```python
from build123d import *

# Parameters (mm, degrees)
BOSS_EXTRUDE1_DEPTH      = 3
BOSS_EXTRUDE1_DEPTH_BACK = 3
FILLET1_R                = 1


with BuildPart() as part:
    # Sketch2 → Boss-Extrude1 (new body, two sides)
    with BuildSketch(Plane(origin=(58.083917136, 121.431989422, 69.518693427), x_dir=(0.999322072, -0.036815702, 0), z_dir=(0, 0, 1))) as boss_extrude1_sk:
        with BuildLine():
            ThreePointArc((18.431354186, -334.485007307), (12.322654185, -340.593707309), (6.213954184, -334.485007307))
            Line((6.213954184, -334.485007307), (-8.62450673, -0.768484104))
            ThreePointArc((-8.62450673, -0.768484104), (-8.650130074, -0.384621702), (-8.658676813, 0))
            ThreePointArc((-8.658676813, 0), (0, 8.658676813), (8.658676813, 0))
            Line((8.658676813, 0), (21.001241455, -149.039780561))
            Line((21.001241455, -149.039780561), (21.131937197, -152.587373918))
            Line((21.131937197, -152.587373918), (18.13397098, -152.697821023))
            Line((18.13397098, -152.697821023), (18.003275238, -149.150227667))
            Line((18.003275238, -149.150227667), (17.003953166, -149.187043369))
            Line((17.003953166, -149.187043369), (17.17146461, -153.733958797))
            Line((17.17146461, -153.733958797), (22.168074971, -153.549880288))
            Line((22.168074971, -153.549880288), (22.00294469, -149.067598925))
            Line((22.00294469, -149.067598925), (9.66, 0))
            ThreePointArc((9.66, 0), (0, 9.66), (-9.66, 0))
            Line((-9.66, 0), (-9.621878236, -0.857355938))
            Line((-9.621878236, -0.857355938), (5.212654184, -334.485007307))
            ThreePointArc((5.212654184, -334.485007307), (12.322654185, -341.595007309), (19.432654186, -334.485007307))
            Line((19.432654186, -334.485007307), (24.411992001, -214.458560592))
            Line((24.411992001, -214.458560592), (24.244480558, -209.911645163))
            Line((24.244480558, -209.911645163), (19.247192269, -210.095748648))
            Line((19.247192269, -210.095748648), (19.414703712, -214.642664077))
            Line((19.414703712, -214.642664077), (20.414703712, -214.605823399))
            Line((20.414703712, -214.605823399), (20.284007971, -211.058230043))
            Line((20.284007971, -211.058230043), (23.281974187, -210.947782937))
            Line((23.281974187, -210.947782937), (23.412669929, -214.495376294))
            Line((23.412669929, -214.495376294), (18.431354186, -334.485007307))
        make_face()
    extrude(amount=BOSS_EXTRUDE1_DEPTH)
    extrude(boss_extrude1_sk.sketch, amount=-BOSS_EXTRUDE1_DEPTH_BACK)

    # Fillet1
    fillet1_edges = [part.edges().sort_by_distance(p)[0] for p in [
        (74.583917136, -32.829928381, 69.518693427),
        (69.583917136, -32.829928381, 69.518693427),
        (69.583238749, -89.229928381, 69.518693427),
        (74.583917136, -89.229928381, 69.518693427),
    ]]
    fillet(fillet1_edges, radius=FILLET1_R)


solid = part.part
```
Input: part model. Units: mm. Frame: model coordinates. A direction names the side the tool comes from. Give positions to 0.01 mm unless a question says otherwise; leave off trailing zeros. Write each loop counter-clockwise with the first axis right and the second up, starting at its lowest first coordinate (ties: lowest second). Pieces come first, ordered by that corner, then holes. Notation, with made-up numbers: (82.25, 47.25) - (95.25, 47.25) arc R9 cw to (95.25, 52.25) - close; hole circle Ø9 at (89.25, -39.75). An arc over 180 degrees is marked (long way). Write item = value, one per line. Start each with the question number.
1) Reachability of faces 4 (the face through (70.112, 47.462, 69.561)), 5 (the face through (50, -44, 72.519)) from +Z, -Z, +X, -X, +Y, -Y: full face, straight path, thin tool, end or side. Return the list, or none.
2) Cut plane A-A (y = -10). Return loops of the section in (x, z), and give its area (3 significant figures).
3) Draft query along X for faces 1 (the face through (57.666, -220.378, 69.561)), 2 (the face through (57.993, -219.388, 69.561)), 3 (the face through (69.82, -154.5, 69.56)). Return one class per face: pulls with the +X half, pulls with the -X half, needs draft (parallel to the pull), parting line crosses it, or undercut.
4) Cut plane C-C (z = 71.1). Return loops of the section in (x, y), and give its area (3 significant figures).
5) Pin query (flat end, axial travel): pin 1 (3 mm diameter, centred on y = -30, z = 71, fed in from -X); pin 2 (2 mm diameter, centred on y = -114.5, z = 69, fed in from -X); pin 3 (12 mm diameter, centred on x = 68.5, y = 37, fed in from -Z); pin 4 (1.8 mm diameter, centred on y = -91.5, z = 70, fed in from -X). Return the tip coordinate at first contact, or that it passes through.
6) Material intervals for L1, parallel to Y at x = 57.75, z = 68.35; L2, parallel to Y at x = 62.25, z = 68.9; L3, parallel to X at y = -166.5, z = 69.8, sorted ascending. Write a range as [from, to].
7) Cut plane B-B (x = 58.25). Return loops of the section in (y, z).
Answers follow:
q1.face_4 = +Z, -Z
q1.face_5 = +Z, +X, -X, +Y, -Y
q2.outline = (49.43, 66.52) - (50.43, 66.52) - (50.43, 72.52) - (49.43, 72.52) - close; (72.75, 66.52) - (73.74, 66.52) - (73.74, 72.52) - (72.75, 72.52) - close
q2.area = 12.0 mm^2
q3.face_1 = parting line crosses it
q3.face_2 = undercut
q3.face_3 = pulls with the +X half
q4.outline = (48.43, 121.79) - (50.98, -213.02) arc R7.11 ccw to (65.19, -213.54) - (74.58, -93.78) - (74.58, -90.23) arc R1 ccw to (73.58, -89.23) - (70.58, -89.23) arc R1 ccw to (69.58, -90.23) - (69.58, -93.78) - (70.58, -93.78) - (70.58, -90.23) - (73.58, -90.23) - (73.58, -93.78) - (64.19, -213.5) arc R6.11 cw to (51.98, -213.06) - (49.44, 120.98) arc R8.66 cw (long way) to (66.74, 121.11) - (73.58, -28.28) - (73.58, -31.83) - (70.58, -31.83) - (70.58, -28.28) - (69.58, -28.28) - (69.58, -31.83) arc R1 ccw to (70.58, -32.83) - (73.58, -32.83) arc R1 ccw to (74.58, -31.83) - (74.58, -28.34) - (67.74, 121.08) arc R9.66 ccw to start
q4.area = 677 mm^2
q5.pin_1 = 49.57
q5.pin_2 = 50.22
q5.pin_3 = 66.52
q5.pin_4 = 50.05
q6.L1 = [-220.38, -219.38], [130.08, 131.09]
q6.L2 = [-219.04, -217.75], [129.02, 130.15]
q6.L3 = [50.62, 51.63], [67.88, 68.88]
q7.outline = (-220.39, 66.52) - (-219.39, 66.52) - (-219.39, 72.52) - (-220.39, 72.52) - close; (130.09, 66.52) - (131.09, 66.52) - (131.09, 72.52) - (130.09, 72.52) - close
